For this review, take the finished solid that the model builds, in its own axes (mm). Face numbers are marked on the shaded views. A direction names the side the tool comes from. Round coordinates to 2 decimals unless told otherwise and drop trailing zeros. Loops run counter-clockwise (first coordinate to the right, second up) from the corner with the lowest first, then second, coordinate; pieces in that order, holes last. Notation, with made-up numbers: M 14,89 L 55,89 A15 cw 55,95 Z; hole C 17,-38.5 d7. An arc over 180 degrees is marked long. One line per question, with ' | ' between items. Start each with the question number.
1) We need section C-C (y = -81.5). Give the boundary of the cut face in (x, z).
2) We need section A-A (z = 0). State how many separate pieces and enclosed holes the cut face has, and give its area (3 significant figures).
3) For the marked faces 1 and 2, list the 3-axis set-ups (+Z, -Z, +X, -X, +Y, -Y) from which the entire face can be reached by the end or side of a thin tool; tool diameter is ignored.
4) For pin 1 Ø2 at (x, z) = (-9.5, 18.5) entering from +Y, flat-tipped, find the tip position at first contact; note if it passes through.
5) For probe 1 along X at (y, z) = (84, -2.5); probe 2 along X at (y, z) = (79, -17.5), list the stretches that pass through material, from the lowest coordinate up. Write a range as from..to.
6) Mouldability with a two-part tool opening along Z and no side actions: class the marked faces 3, 4 and 5 as pulls with the +Z half, pulls with the -Z half, needs draft (parallel to the pull), parting line crosses it, or undercut.
7) We need section B-B (x = 4.5). Give the boundary of the cut face in (y, z).
```python
from build123d import *

# Parameters (mm, degrees)
F0_W     = 50.8
F0_H     = 50.8
F0_W_2   = 41.275
F0_H_2   = 41.275
F1_DEPTH = 171.45
F2_R     = 5.08
F3_R     = 6.35
F4_DEPTH = 50.801


with BuildPart() as f1:
    # F0 (on Front) → F1 (new body, symmetric)
    with BuildSketch(Plane.XZ):
        Rectangle(F0_W, F0_H)
        Rectangle(F0_W_2, F0_H_2, mode=Mode.SUBTRACT)
    extrude(amount=F1_DEPTH, both=True)

    # F2
    f2_edges = [f1.edges().sort_by_distance(p)[0] for p in [
        (-20.6375, 0, 20.6375),
        (25.4, 0, -25.4),
        (-25.4, 0, -25.4),
        (25.4, 0, 25.4),
        (20.6375, 0, -20.6375),
        (-25.4, 0, 25.4),
        (20.6375, 0, 20.6375),
        (-20.6375, 0, -20.6375),
    ]]
    fillet(f2_edges, radius=F2_R)

    # F3 (on face) → F4 (cut, through all)
    with BuildSketch(Plane.YZ.offset(25.4)):
        with Locations((-155.575, 0)):
            Circle(F3_R)
        with Locations((155.575, 0)):
            Circle(F3_R)
    extrude(amount=-F4_DEPTH, mode=Mode.SUBTRACT)


solid = f1.part
```
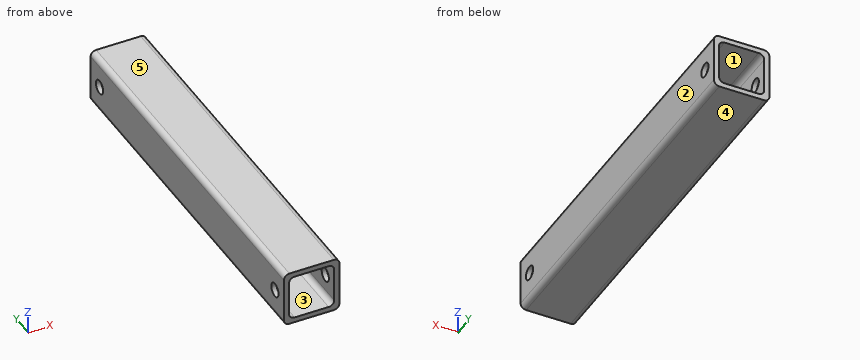
Answers below:
1) outline: M -25.4,-20.32 A5.08 ccw -20.32,-25.4 L 20.32,-25.4 A5.08 ccw 25.4,-20.32 L 25.4,20.32 A5.08 ccw 20.32,25.4 L -20.32,25.4 A5.08 ccw -25.4,20.32 Z; hole M -20.64,-15.56 A5.08 ccw -15.56,-20.64 L 15.56,-20.64 A5.08 ccw 20.64,-15.56 L 20.64,15.56 A5.08 ccw 15.56,20.64 L -15.56,20.64 A5.08 ccw -20.64,15.56 Z
2) separate pieces: 6 | enclosed holes: 0 | area: 3,020 mm^2
3) face 1: +Y, -Y | face 2: +Z, -Z, +X, +Y, -Y
4) pin 1: through
5) probe 1: -25.4..-20.64, 20.64..25.4 | probe 2: -25.4..-20.25, 20.25..25.4
6) face 3: undercut | face 4: pulls with the -Z half | face 5: pulls with the +Z half
7) outline: M -171.45,-25.4 L 171.45,-25.4 L 171.45,-20.64 L -171.45,-20.64 Z; M -171.45,20.64 L 171.45,20.64 L 171.45,25.4 L -171.45,25.4 Z
